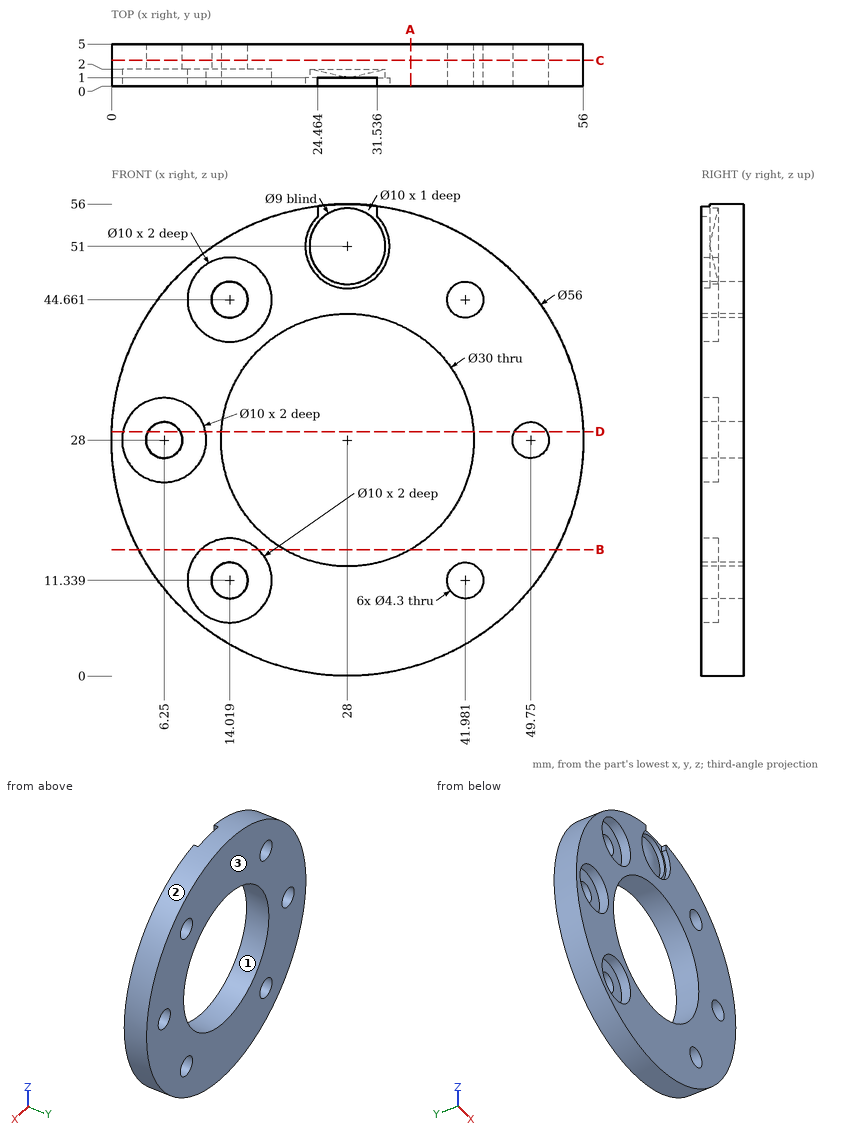
Print and shaded views of the part. All mm, measured from the part's lowest x, y and z. Give positions to 0.01 mm unless a question says otherwise; leave off trailing zeros. Order: outer loops, then holes, each group sorted by start corner. A loop starts at its lowest first (then second) coordinate and runs counter-clockwise, first axis right, second up. Notation, with made-up numbers: (13, -9) -> (36, -9) arc R28 ccw to (36, 11) -> close; hole circle Ø5 at (71.5, -29). An arc over 180 degrees is marked (long way). Use CSV: the item, a comma, the result in double quotes.
1. Mould opens along X. For the marked faces 1, 2 and 3 say: +X half, -X half, draft (parallel to the pull), parting line (faces both ways), or undercut.
Outcome:
face 1,"undercut"
face 2,"parting line"
face 3,"draft"
2. Drop flat-ended pins along their axis: pin 1 (13 mm diameter, centred on x = 6.25, z = 28, fed in from -Y); pin 2 (5 mm diameter, centred on x = 14.02, z = 11.34, fed in from -Y); pin 3 (3 mm diameter, centred on x = 30, z = 51, fed in from -Y). Give the stop position or say it passes through.
Outcome:
pin 1,"y = 0"
pin 2,"y = 2"
pin 3,"y = 1.11"
3. Band-saw the part on C-C, the plane y = 3.05. Give the cut face in (x, z), then the cut area to 3 significant figures.
Outcome:
outline,"circle Ø56 at (28, 28); hole circle Ø4.3 at (6.25, 28); hole circle Ø4.3 at (14.02, 11.34); hole circle Ø4.3 at (14.02, 44.66); hole circle Ø30 at (28, 28); hole circle Ø4.3 at (41.98, 11.34); hole circle Ø4.3 at (41.98, 44.66); hole circle Ø4.3 at (49.75, 28)"
area,"1,670 mm²"
4. Band-saw the part on A-A, the plane x = 35.5. Give the cut face in (y, z).
Outcome:
outline,"(0, 1.02) -> (5, 1.02) -> (5, 15.01) -> (0, 15.01) -> close; (0, 40.99) -> (5, 40.99) -> (5, 54.98) -> (0, 54.98) -> close"
5. Drill centre lines: line 1 along X through (y, z) = (4.05, 28); line 2 along Z through (x, y) = (3, 1.15) (1 decimal); line 3 along Z through (x, y) = (37, 3.7) (1 decimal). Where is each one in solid material? Low to high. Write a range as from..to.
Outcome:
line 1,"0..4.1, 8.4..13, 43..47.6, 51.9..56"
line 2,"15.4..24.2, 31.8..40.6"
line 3,"1.5..16, 40..54.5"
6. Band-saw the part on B-B, the plane z = 15. Give the cut face in (x, y) (1 decimal).
Outcome:
outline,"(3.2, 0) -> (10.6, 0) -> (10.6, 2) -> (17.4, 2) -> (17.4, 0) -> (20.5, 0) -> (20.5, 5) -> (3.2, 5) -> close; (35.5, 0) -> (52.8, 0) -> (52.8, 5) -> (35.5, 5) -> close"
7. Band-saw the part on D-D, the plane z = 29. Give the cut face in (x, y).
Outcome:
outline,"(0.02, 0) -> (1.35, 0) -> (1.35, 2) -> (4.35, 2) -> (4.35, 5) -> (0.02, 5) -> close; (8.15, 2) -> (11.15, 2) -> (11.15, 0) -> (13.03, 0) -> (13.03, 5) -> (8.15, 5) -> close; (42.97, 0) -> (47.85, 0) -> (47.85, 5) -> (42.97, 5) -> close; (51.65, 0) -> (55.98, 0) -> (55.98, 5) -> (51.65, 5) -> close"
